```python
from build123d import *

# Parameters (mm, degrees)
F1_W     = 63.0000010133
F1_H     = 98.0000010133
F2_DEPTH = 16
F0_W     = 60
F0_H     = 95
F3_DEPTH = 14
F4_R     = 5
F5_R     = 1.5


with BuildPart() as f2:
    # F1 (on Top) → F2 (new body)
    with BuildSketch(Plane.XY):
        Rectangle(F1_W, F1_H)
    extrude(amount=F2_DEPTH)

    # F0 (on Top) → F3 (cut, through all)
    with BuildSketch(Plane.XY):
        Rectangle(F0_W, F0_H)
    extrude(amount=F3_DEPTH, mode=Mode.SUBTRACT)

    # F4
    f4_edges = [f2.edges().sort_by_distance(p)[0] for p in [
        (-30, 47.5, 7),
        (30, 47.5, 7),
        (31.500001, 49.000001, 8),
        (-31.500001, 49.000001, 8),
        (-31.500001, -49.000001, 8),
        (-30, -47.5, 7),
        (30, -47.5, 7),
        (31.500001, -49.000001, 8),
    ]]
    fillet(f4_edges, radius=F4_R)

    # F5
    f5_edges = [f2.edges().sort_by_distance(p)[0] for p in [
        (0, 49.000001, 16),
        (30.035534, 47.535534, 16),
        (-30.035534, 47.535534, 16),
        (31.500001, 0, 16),
        (-31.500001, 0, 16),
        (30.035534, -47.535534, 16),
        (-30.035534, -47.535534, 16),
        (0, -49.000001, 16),
    ]]
    fillet(f5_edges, radius=F5_R)

    # F8: sweep along a path in F6
    with BuildLine(Plane.XY) as f8_path:
        Line((25, -47.5), (-25, -47.5))
        ThreePointArc((-25, -47.5), (-28.5355339059, -46.0355339059), (-30, -42.5))
        Line((-30, -42.5), (-30, 42.5))
        ThreePointArc((-30, 42.5), (-28.5355339059, 46.0355339059), (-25, 47.5))
        Line((-25, 47.5), (25, 47.5))
        ThreePointArc((25, 47.5), (28.5355339059, 46.0355339059), (30, 42.5))
        Line((30, 42.5), (30, -42.5))
        ThreePointArc((30, -42.5), (28.5355339059, -46.0355339059), (25, -47.5))
    # F7 (on Front) → F8 (sweep)
    with BuildSketch(Plane.XZ):
        with BuildLine():
            ThreePointArc((-29, -1), (-29.7071067812, -0.7071067812), (-30, 0))
            Line((-30, 0), (-31.5000005066, 0))
            Line((-31.5000005066, 0), (-31.5000005066, -1))
            Line((-31.5000005066, -1), (-30, -1))
            Line((-30, -1), (-29, -1))
        make_face()
    sweep(path=f8_path.line)


solid = f2.part
```
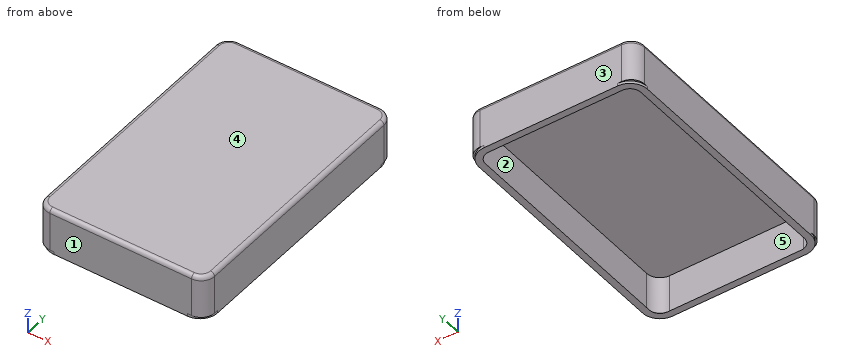
Here's how the part is built. I have some questions about the finished solid (model axes, mm). Face numbers are marked on the shaded views. A direction names the side the tool comes from. Give positions to 0.01 mm unless a question says otherwise; leave off trailing zeros. Loops run counter-clockwise (first coordinate to the right, second up) from the corner with the lowest first, then second, coordinate; pieces in that order, holes last. Notation, with made-up numbers: M -23.75,-40 L 26.25,-40 A7 ccw 26.25,-35 Z; hole C 72,-22.5 d7. An arc over 180 degrees is marked long. Return JSON: item names as keys, results as strings.
Item 1: Thinking about a two-plate mould opening in Z: for the marked faces 3, 4 and 5, which applies, released by +Z, released by -Z, zero draft, split by the parting line, or undercut?
A:
{"face 3": "zero draft", "face 4": "released by +Z", "face 5": "undercut"}
Item 2: Imagine slicing it at B-B on x = 22.5. List the corners of the cut face in (y, z) for me, then the cut area to 3 significant figures.
A:
{"outline": "M -49,-1 L -46.5,-1 A1 cw -47.5,0 L -47.5,14 L 47.5,14 L 47.5,0 A1 cw 46.5,-1 L 49,-1 L 49,14.5 A1.5 ccw 47.5,16 L -47.5,16 A1.5 ccw -49,14.5 Z", "area": "240 mm^2"}
Item 3: Imagine slicing it at C-C on y = -25. List the corners of the cut face in (x, z) for me, then the cut area to 3 significant figures.
A:
{"outline": "M -31.5,-1 L -29,-1 A1 cw -30,0 L -30,14 L 30,14 L 30,0 A1 cw 29,-1 L 31.5,-1 L 31.5,14.5 A1.5 ccw 30,16 L -30,16 A1.5 ccw -31.5,14.5 Z", "area": "170 mm^2"}
Item 4: I'm going to push a flat-ended pin straight in: pin 1 Ø3 at (x, y) = (23, 2.5) entering from -Z. Where does the tip first touch, or does it pass through?
A:
{"pin 1": "stops at z = 14"}
Item 5: Please list where these lines run through material, in increasing order: line 1 (X direction, y = 19, z = 11); line 2 (Y direction, x = -3, z = 7.25); line 3 (Z direction, x = 5.5, y = -27).
A:
{"line 1": "x = -31.5 to -30, 30 to 31.5", "line 2": "y = -49 to -47.5, 47.5 to 49", "line 3": "z = 14 to 16"}
Item 6: On a 3-axis mill with a long thin cutter (end or side, diameter ignored), from which of +Z, -Z, +X, -X, +Y, -Y can I reach the whole of each face in a straight line? I mean the marked faces 1 and 2. Say none if no direction works.
A:
{"face 1": "+Z, -Z, +X, -X, -Y", "face 2": "none"}
Item 7: Imagine slicing it at A-A on z = 1. List the corners of the cut face in (x, y) for me, then the cut area to 3 significant figures.
A:
{"outline": "M -31.5,-44 A5 ccw -26.5,-49 L 26.5,-49 A5 ccw 31.5,-44 L 31.5,44 A5 ccw 26.5,49 L -26.5,49 A5 ccw -31.5,44 Z; hole M -30,-42.5 A5 ccw -25,-47.5 L 25,-47.5 A5 ccw 30,-42.5 L 30,42.5 A5 ccw 25,47.5 L -25,47.5 A5 ccw -30,42.5 Z", "area": "474 mm^2"}
